The model under review builds one solid part; all positions refer to its coordinate system, in mm. A direction names the side the tool comes from. Round coordinates to 2 decimals unless told otherwise and drop trailing zeros. Write each loop counter-clockwise with the first axis right and the second up, starting at its lowest first coordinate (ties: lowest second). Pieces come first, ordered by that corner, then holes. Notation, with made-up numbers: M 25.25,2 L 61.25,2 A22 ccw 61.25,15 Z; hole C 63.25,-33.75 d7. An arc over 180 degrees is marked long. Write item = value, one per line. Start each with the question number.
Item 1: For pin 1 Ø1 at (x, y) = (136.5, 0.5) entering from +Z; pin 2 Ø3 at (y, z) = (3, 40) entering from +X; pin 3 Ø1.2 at (y, z) = (4, 84) entering from -X, all flat-tipped, find the tip position at first contact; note any pin that passes through.
Item 2: Take a section at C-C, the plane y = 1.6. Give the boundary of the cut face in (x, z).
Item 3: Tool access review of faces 5 (the flat face through (171, 2.5, 82)), 6 (the flat face through (133, 3, 81.465)), 7 (the flat face through (15, 2.5, 82)), 8 (the flat face through (-6.254, 2, -46)), 9 (the flat face through (-29, 2, -38.535)): name each direction out of +Z, -Z, +X, -X, +Y, -Y from which nothing blocks a thin tool from reaching the whole face with its end or side.
Item 4: Take a section at B-B, the plane x = 169. Give the boundary of the cut face in (y, z), plus the area to 3 significant figures.
Item 5: The part is to be moulded in two halves that separate along Z. For faces 1 (the flat face through (206, 2, 16.465)), 2 (the flat face through (206, 2, 46.465)), 3 (the flat face through (54, 3, 81.465)), 4 (the flat face through (68.746, 2, -46)), say which applies: +Z half, -Z half, draft (parallel to the pull), parting line (faces both ways), or undercut.
Item 6: Take a section at D-D, the plane x = 92.5. Give the boundary of the cut face in (y, z), plus the area to 3 significant figures.
Item 7: To check wall thickness, follow line 1 along Z through (x, y) = (51, 3.8); line 2 along X through (y, z) = (0.95, 38.5); line 3 along X through (y, z) = (0.4, -11). State the ranges of each line that lie inside material, in increasing order.
from build123d import *

# Parameters (mm, degrees)
SKETCH_1_W          = 5
SKETCH_1_H          = 60
SKETCH_1_W_2        = 30
SKETCH_1_H_2        = 5
SKETCH_1_W_3        = 15
EXTRUDE_1_DEPTH     = 5
FILLET_1_R          = 5
SKETCH_2_W          = 239.490005879
SKETCH_2_H          = 213.108485662
CUT_EXTRUDE_2_DEPTH = 10
SKETCH_3_W          = 73
SKETCH_3_H          = 2.5
SKETCH_3_W_2        = 74
CUT_EXTRUDE_3_DEPTH = 10
SKETCH_4_W          = 5
SKETCH_4_H          = 5
CUT_EXTRUDE_4_DEPTH = 5


with BuildPart() as part:
    # 草圖1 → 填料-伸長1 (new body)
    with BuildSketch(Plane(origin=(0, 0, 0), x_dir=(1, 0, 0), z_dir=(0, 1, 0))):
        Polygon((198.746286718, -286.464902661), (198.746286718, -256.464902661), (183.246286718, -256.464902661), (183.246286718, -266.464902661), (124.746286718, -266.464902661), (124.746286718, -262.464902661), (109.246286718, -262.464902661), (109.246286718, -266.464902661), (-21.253713282, -266.464902661), (-21.253713282, 38.535097339), (-36.253713282, 38.535097339), (-36.253713282, 43.535097339), (203.746286718, 43.535097339), (203.746286718, -286.464902661), align=None)
        with Locations((206.246286718, -256.464902661)):
            Rectangle(SKETCH_1_W, SKETCH_1_H)
        with Locations((206.246286718, 13.535097339)):
            Rectangle(SKETCH_1_W, SKETCH_1_H)
        with Locations((188.746286718, 46.035097339)):
            Rectangle(SKETCH_1_W_2, SKETCH_1_H_2)
        with Locations((-21.253713282, 46.035097339)):
            Rectangle(SKETCH_1_W_2, SKETCH_1_H_2)
        with Locations((91.246286718, 46.035097339)):
            Rectangle(SKETCH_1_W_3, SKETCH_1_H_2)
        with Locations((76.246286718, 46.035097339)):
            Rectangle(SKETCH_1_W_3, SKETCH_1_H_2)
        with Locations((206.246286718, -166.464902661)):
            Rectangle(SKETCH_1_W, SKETCH_1_H)
        with Locations((206.246286718, -76.464902661)):
            Rectangle(SKETCH_1_W, SKETCH_1_H)
    extrude(amount=EXTRUDE_1_DEPTH)

    # 圓角1
    fillet_1_edges = [part.edges().sort_by_distance(p)[0] for p in [
        (208.746286718, 5, -13.535097339),
        (208.746286718, 5, 76.464902661),
        (208.746286718, 5, 166.464902661),
        (208.746286718, 5, 256.464902661),
    ]]
    fillet(fillet_1_edges, radius=FILLET_1_R - 0.0001)  # a hair under: the kernel refuses the full size

    # 草圖2 → 除料-伸長2 (cut)
    with BuildSketch(Plane(origin=(0, 5, 0), x_dir=(1, 0, 0), z_dir=(0, 1, 0))):
        with Locations((89.001283779, -193.019145492)):
            Rectangle(SKETCH_2_W, SKETCH_2_H)
    extrude(amount=-CUT_EXTRUDE_2_DEPTH, mode=Mode.SUBTRACT)

    # 草圖3 → 除料-伸長3 (cut)
    with BuildSketch(Plane.XY.offset(86.464902661)):
        with Locations((15.246286718, 1.25)):
            Rectangle(SKETCH_3_W, SKETCH_3_H)
        with Locations((172.246286718, 1.25)):
            Rectangle(SKETCH_3_W, SKETCH_3_H)
        with Locations((93.746286718, 3.75)):
            Rectangle(SKETCH_3_W_2, SKETCH_3_H)
    extrude(amount=-CUT_EXTRUDE_3_DEPTH, mode=Mode.SUBTRACT)

    # 草圖4 → 除料-伸長4 (cut)
    with BuildSketch(Plane.XY.offset(86.464902661)):
        with Locations((54.246286718, 2.5)):
            Rectangle(SKETCH_4_W, SKETCH_4_H)
        with Locations((133.246286718, 2.5)):
            Rectangle(SKETCH_4_W, SKETCH_4_H)
    extrude(amount=-CUT_EXTRUDE_4_DEPTH, mode=Mode.SUBTRACT)


solid = part.part
Response values:
q1.pin_1 = 76.46
q1.pin_2 = 203.75
q1.pin_3 = -21.25
q2.outline = M -36.25,-48.54 L -6.25,-48.54 L -6.25,-43.54 L 68.75,-43.54 L 68.75,-48.54 L 98.75,-48.54 L 98.75,-43.54 L 173.75,-43.54 L 173.75,-48.54 L 203.75,-48.54 L 203.75,-43.54 L 208.48,-43.54 L 208.48,16.46 L 203.75,16.46 L 203.75,46.46 L 208.48,46.46 L 208.48,76.46 L 135.75,76.46 L 135.75,81.46 L 130.75,81.46 L 130.75,86.46 L 56.75,86.46 L 56.75,81.46 L 51.75,81.46 L 51.75,76.46 L -21.25,76.46 L -21.25,-38.54 L -36.25,-38.54 Z
q3.face_5 = +Z, +X, -Y
q3.face_6 = +Z, +Y, -Y
q3.face_7 = +Z, -X, -Y
q3.face_8 = -Z, +Y, -Y
q3.face_9 = +Z, -X, +Y, -Y
q4.outline = M 0,-43.54 L 5,-43.54 L 5,86.46 L 2.5,86.46 L 2.5,76.46 L 0,76.46 Z
q4.area = 625 mm2
q5.face_1 = undercut
q5.face_2 = undercut
q5.face_3 = +Z half
q5.face_4 = draft
q6.outline = M 0,-48.54 L 5,-48.54 L 5,76.46 L 2.5,76.46 L 2.5,86.46 L 0,86.46 Z
q6.area = 650 mm2
q7.line_1 = -43.54 to 86.46
q7.line_2 = -21.25 to 203.75
q7.line_3 = -21.25 to 208.73
